from build123d import *

# Parameters (mm, degrees)
F1_DEPTH = 63.5
F2_DEPTH = 25.4
F3_DEPTH = 7.9375
F0_W     = 14.291249726
F0_H     = 4.7752
F0_H_2   = 4.7498
F0_H_3   = 19.05
F5_R     = 5.08


with BuildPart() as f1:
    # F0 (on Front) → F1 (new body, symmetric)
    with BuildSketch(Plane.XZ):
        Polygon((22.225, 9.525), (-41.275, 9.525), (-41.275, -9.525), (41.275, -9.525), (41.275, 9.525), align=None)
    extrude(amount=F1_DEPTH, both=True)

    # F0 (on Front) → F2 (join, symmetric)
    with BuildSketch(Plane.XZ):
        with BuildLine():
            Line((22.225, 27.0002), (22.225, 9.525))
            Line((22.225, 9.525), (41.275, 9.525))
            Line((41.275, 9.525), (41.275, 27.0002))
            ThreePointArc((41.275, 27.0002), (45.9246798487, 38.2255201513), (57.15, 42.8752))
            Line((57.15, 42.8752), (71.433750274, 42.8752))
            Line((71.433750274, 42.8752), (71.433750274, 61.9252))
            Line((71.433750274, 61.9252), (67.8752437234, 61.9252))
            Line((67.8752437234, 61.9252), (63.7876612968, 61.9252))
            add(Edge.make_bspline(
                [(52.4566688637, 61.6084109888), (56.1143116658, 61.7901051123), (59.8906472041, 61.8974539816), (63.7876612968, 61.9252)],
                knots=[112.7369449664, 112.7369449664, 112.7369449664, 112.7369449664, 118.9332301847, 118.9332301847, 118.9332301847, 118.9332301847], degree=3))
            ThreePointArc((52.4566688637, 61.6084109888), (30.8472414476, 49.9767210059), (22.225, 27.0002))
        make_face()
    extrude(amount=F2_DEPTH, both=True)

    # F0 (on Front) → F3 (join, symmetric)
    with BuildSketch(Plane.XZ):
        with BuildLine():
            add(Edge.make_bspline(
                [(-41.275, 9.525), (-41.3486110715, 30.3861799307), (-14.0915064954, 58.3026173271), (52.4566688637, 61.6084109888)],
                knots=[0, 0, 0, 0, 112.7369449664, 112.7369449664, 112.7369449664, 112.7369449664], degree=3))
            Line((-41.275, 9.525), (22.225, 9.525))
            Line((22.225, 9.525), (22.225, 27.0002))
            ThreePointArc((22.225, 27.0002), (30.8472414476, 49.9767210059), (52.4566688637, 61.6084109888))
        make_face()
    extrude(amount=F3_DEPTH, both=True)

    # F0 (on Front) → F4 (revolve)
    with BuildSketch(Plane.XZ):
        with Locations((78.579375137, 40.4876)):
            Rectangle(F0_W, F0_H)
        with Locations((78.579375137, 64.3001)):
            Rectangle(F0_W, F0_H_2)
        with Locations((78.579375137, 52.4002)):
            Rectangle(F0_W, F0_H_3)
        Polygon((85.725, 66.675), (85.725, 61.9252), (85.725, 42.8752), (85.725, 38.1), (122.233750274, 38.1), (122.233750274, 66.675), align=None)
    revolve(axis=Axis((71.433750274, 0, 52.3875), (0, 0, -1)))

    # F5
    f5_edges = [f1.edges().sort_by_distance(p)[0] for p in [
        (41.275, -63.5, 0),
        (-41.275, -63.5, 0),
        (41.275, 63.5, 0),
        (-41.275, 63.5, 0),
    ]]
    fillet(f5_edges, radius=F5_R)


solid = f1.part
Design review of the part built by this model. Coordinates are the model's own, in mm. A direction names the side the tool comes from. Coordinates: 2 decimals unless noted, no trailing zeros. Order: outer loops, then holes, each group sorted by start corner. A loop starts at its lowest first (then second) coordinate and runs counter-clockwise, first axis right, second up. Notation, with made-up numbers: M 86,-36.5 L 104,-36.5 A17 cw 104,-15.5 Z; hole C 72.5,34 d1. An arc over 180 degrees is marked long. Use a Markdown table: item, result.
(1) Add section B-B (z = 2). Give the boundary of the cut face in (x, y) (3 decimals).
Worked answers:
| item | result |
|---|---|
| outline | M -41.275,-58.42 A5.08 ccw -36.195,-63.5 L 36.195,-63.5 A5.08 ccw 41.275,-58.42 L 41.275,58.42 A5.08 ccw 36.195,63.5 L -36.195,63.5 A5.08 ccw -41.275,58.42 Z |
(2) Add section C-C (y = -32.5). Give the boundary of the cut face in (x, z) (3 decimals).
Worked answers:
| item | result |
|---|---|
| outline | M -41.275,-9.525 L 41.275,-9.525 L 41.275,9.525 L -41.275,9.525 Z; M 32.39,38.1 L 110.477,38.1 L 110.477,66.675 L 32.39,66.675 Z |
(3) Add section D-D (y = -16.5). Give the boundary of the cut face in (x, z) (3 decimals), then the cut area to 3 significant figures.
Worked answers:
| item | result |
|---|---|
| outline | M -41.275,-9.525 L 41.275,-9.525 L 41.275,27 A15.875 cw 45.801,38.1 L 119.479,38.1 L 119.479,66.675 L 23.388,66.675 L 23.388,38.1 L 24.036,38.1 A34.925 ccw 22.225,27 L 22.225,9.525 L -41.275,9.525 Z |
| area | 4,870 mm2 |
(4) Wall thickness on probe 1 along Y at (x, z) = (20, 29); probe 2 along Z at (x, y) = (81, -35) (3 decimals); probe 3 along Z at (x, y) = (-12.5, 55) (3 decimals): over which ranges is each line inside the solid? List them lowest first.
Worked answers:
| item | result |
|---|---|
| probe 1 | y = -7.94 to 7.94 |
| probe 2 | z = 38.1 to 66.675 |
| probe 3 | z = -9.525 to 9.525 |
(5) For faces 1 (the flat face through (41.275, -1, 4)), 2 (the cylindrical face through (-39.8, -62, -0.1)), 3 (the flat face through (22.225, 17, 18)), list the 3-axis set-ups (+Z, -Z, +X, -X, +Y, -Y) from which the entire face can be reached by the end or side of a thin tool; tool diameter is ignored.
Worked answers:
| item | result |
|---|---|
| face 1 | -Z, +X, +Y, -Y |
| face 2 | +Z, -Z, -X, -Y |
| face 3 | -X, +Y |
(6) Add section A-A (y = -49). Give the boundary of the cut face in (x, z) (3 decimals), then the cut area to 3 significant figures.
Worked answers:
| item | result |
|---|---|
| outline | M -41.275,-9.525 L 41.275,-9.525 L 41.275,9.525 L -41.275,9.525 Z; M 58.031,38.1 L 84.837,38.1 L 84.837,66.675 L 58.031,66.675 Z |
| area | 2,340 mm2 |
(7) For P1, Ø8.5, axis at y = -13.5, z = 15.5, coming from the -X side (3 decimals); P2, Ø5, axis at x = 25, y = -37, coming from the +Z side (3 decimals); P3, Ø7, axis at x = 36.5, z = 36.5, coming from the +Y side, all flat-tipped, find the tip position at first contact; note any pin that passes through.
Worked answers:
| item | result |
|---|---|
| P1 | stops at x = 22.225 |
| P2 | stops at z = 9.525 |
| P3 | stops at y = 39.6 |
